```python
from build123d import *

# Parameters (mm, degrees)
SKETCH2_R               = 4.75
SKETCH3_R               = 4.75
SKETCH4_W               = 2
SKETCH4_H               = 5
BOSS_EXTRUDE1_DEPTH     = 55
SKETCH3_7_W             = 10
SKETCH3_7_H             = 10
BOSS_EXTRUDE4_DEPTH     = 4
SKETCH8_W               = 2
SKETCH8_H               = 8
CUT_EXTRUDE2_DEPTH      = 1
CUT_EXTRUDE2_DEPTH_BACK = 11


with BuildPart() as part:
    # Sketch2 → Loft1 section 0
    with BuildSketch(Plane.XY):
        Circle(SKETCH2_R)
    # Sketch3 → Loft1 section 1
    with BuildSketch(Plane.XY.offset(16.5)):
        Circle(SKETCH3_R)
    loft()

    # Sketch4 → Boss-Extrude1 (add)
    with BuildSketch(Plane(origin=(0, 0, 0), x_dir=(1, 0, 0), z_dir=(0, 1, 0))):
        with Locations((0, -9.5)):
            Rectangle(SKETCH4_W, SKETCH4_H)
    extrude(amount=-BOSS_EXTRUDE1_DEPTH)

    # Sketch3<7> → Boss-Extrude4 (add)
    with BuildSketch(Plane.XY.offset(16.5)):
        Rectangle(SKETCH3_7_W, SKETCH3_7_H)
    extrude(amount=BOSS_EXTRUDE4_DEPTH)

    # Sketch8 → Cut-Extrude2 (cut, two sides)
    with BuildSketch(Plane(origin=(5, 0, 0), x_dir=(0, 0, -1), z_dir=(1, 0, 0))) as cut_extrude2_sk:
        with Locations((-18.5, 0)):
            Rectangle(SKETCH8_W, SKETCH8_H)
    extrude(amount=CUT_EXTRUDE2_DEPTH, mode=Mode.SUBTRACT)
    extrude(cut_extrude2_sk.sketch, amount=-CUT_EXTRUDE2_DEPTH_BACK, mode=Mode.SUBTRACT)


solid = part.part
```
Verification items for the finished model (mm, model axes). A direction names the side the tool comes from. Coordinates: 2 decimals unless noted, no trailing zeros. Write each loop counter-clockwise with the first axis right and the second up, starting at its lowest first coordinate (ties: lowest second). Pieces come first, ordered by that corner, then holes. Notation, with made-up numbers: (-37, -1) - (-28, -1) arc R17 cw to (-28, 5) - close; hole circle Ø6 at (22.5, 3). An arc over 180 degrees is marked (long way). Write item = value, one per line.
Q1. Mould release check, pull along Y, two halves, no side actions. Record for faces 1 (the face through (0, -55, 9)), 2 (the face through (0, -29, 12)), 3 (the face through (0, 0, 17.5)): released by +Y, released by -Y, zero draft, split by the parting line, or undercut.
Answer:
face_1 = released by -Y
face_2 = zero draft
face_3 = undercut
Q2. Cross-section at C-C (z = 1.75). Enter the section's corners in (x, y).
Answer:
outline = circle Ø9.5 at (0, 0)
Q3. Material ranges on L1, parallel to Y at x = -2, z = 17.75; L2, parallel to Z at x = -0.75, y = -9.5; L3, parallel to Z at x = 0.75, y = -1, recorded low to high. Write a range as from..to.
Answer:
L1 = -5..-4, 4..5
L2 = 7..12
L3 = 0..17.5, 19.5..20.5
Q4. Go/stop test with flat-tipped pins: pin 1 Ø2.5 at (y, z) = (-30.5, 10) entering from -X; pin 2 Ø1 at (x, z) = (0.5, 18.5) entering from -Y; pin 3 Ø1.6 at (x, y) = (0.5, -30) entering from +Z. Record where each tip stops, or that it passes through.
Answer:
pin_1 = -1
pin_2 = -5
pin_3 = 12
Q5. Cross-section at D-D (y = -43.5). Enter the section's corners in (x, z), plus the area to 3 significant figures.
Answer:
outline = (-1, 7) - (1, 7) - (1, 12) - (-1, 12) - close
area = 10.0 mm²
Q6. Cross-section at A-A (x = 0). Enter the section's corners in (y, z), plus the area to 3 significant figures.
Answer:
outline = (-55, 7) - (-4.75, 7) - (-4.75, 0) - (4.75, 0) - (4.75, 16.5) - (5, 16.5) - (5, 20.5) - (-5, 20.5) - (-5, 16.5) - (-4.75, 16.5) - (-4.75, 12) - (-55, 12) - close; hole (-4, 17.5) - (4, 17.5) - (4, 19.5) - (-4, 19.5) - close
area = 432 mm²
Q7. Cross-section at B-B (y = -2). Enter the section's corners in (x, z), plus the area to 3 significant figures.
Answer:
outline = (-5, 16.5) - (-4.31, 16.5) - (-4.31, 0) - (4.31, 0) - (4.31, 16.5) - (5, 16.5) - (5, 17.5) - (-5, 17.5) - close; (-5, 19.5) - (5, 19.5) - (5, 20.5) - (-5, 20.5) - close
area = 162 mm²
Q8. Access from +Z, -Z, +X, -X, +Y, -Y to the whole of each face (thin tool, end or side, straight path). Record for faces 4 (the face through (0, -29, 7)), 5 (the face through (1, -29, 10)), 6 (the face through (0, -4, 19)).
Answer:
face_4 = -Z, +X, -X, -Y
face_5 = +Z, -Z, +X, -Y
face_6 = +X, -X
